Input: dimensioned drawing with shaded views. Units: mm. Origin: part minimum x, y, z. Give positions to 0.01 mm unless a question says otherwise; leave off trailing zeros. Loops run counter-clockwise (first coordinate to the right, second up) from the corner with the lowest first, then second, coordinate; pieces in that order, holes last. Notation, with made-up numbers: (52, -26) -> (106, -26) arc R19 cw to (106, -3) -> close; hole circle Ø11 at (-31.5, 21.25). An arc over 180 degrees is marked (long way). Answer in a Markdown table with one row per item. Add a question column.
1) First-contact query: P1, Ø1.5, axis at y = 12, z = 20, coming from the +X side; P2, Ø0.9, axis at x = 17, z = 28, coming from the -Y side; P3, Ø1, axis at x = 17, z = 9.5, coming from the +Y side. Flat tips, straight axial feed; report the tip coordinate or a pass-through.
2) Line query: line 1 (X direction, y = 15, z = 17) (3 decimals); line 2 (X direction, y = 1.75, z = 16.8); line 3 (X direction, y = 5.25, z = 18). Output: solid intervals per line, ascending. Write a range as from..to.
3) Section query C-C (y = 2). Return the cut outline in (x, z), plus the area to 3 significant figures.
4) Section query A-A (x = 16.8). Return the cut outline in (y, z).
5) Section query D-D (z = 28.05). Return the cut outline in (x, y), plus the area to 3 significant figures.
6) Section query B-B (z = 16.8). Return the cut outline in (x, y), plus the area to 3 significant figures.
7) Draft query along X for the marked faces 1, 2 and 3. Return one class per face: +X half, -X half, draft (parallel to the pull), parting line (faces both ways), or undercut.
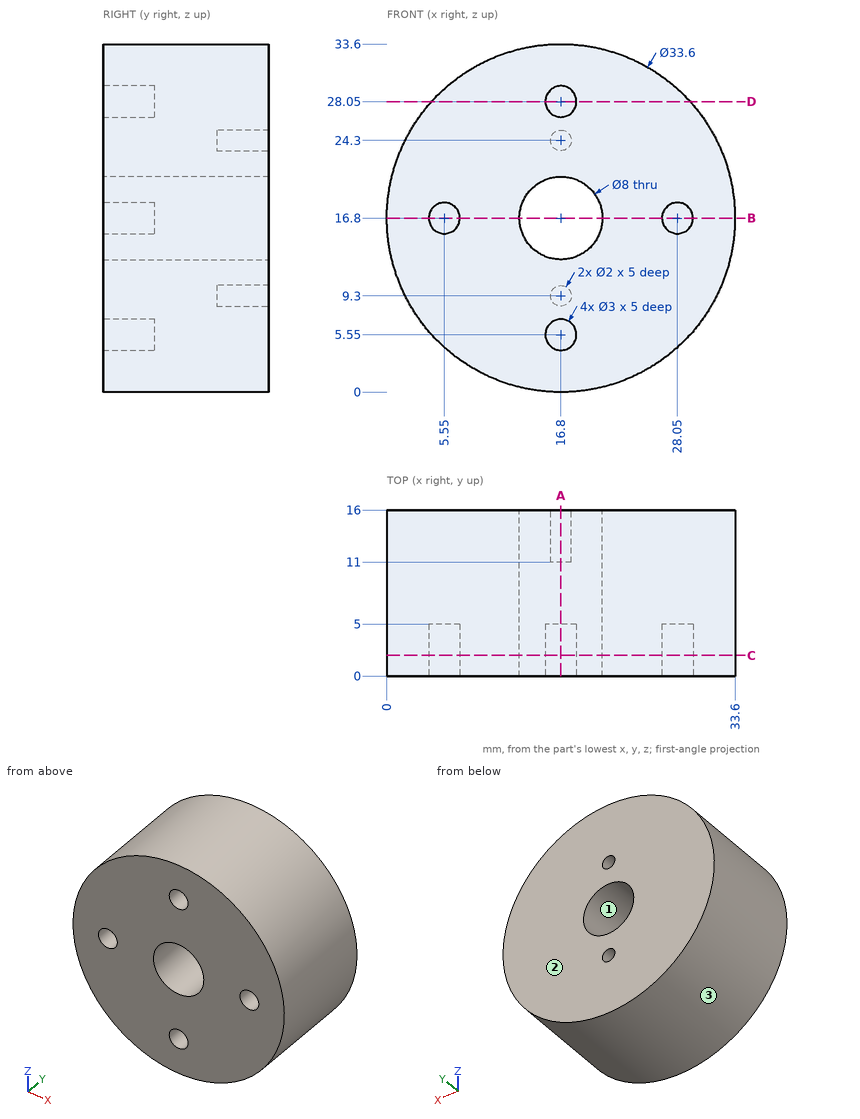
Evaluation:
| question | item | result |
|---|---|---|
| 1 | P1 | x = 33.42 |
| 1 | P2 | y = 5 |
| 1 | P3 | y = 11 |
| 2 | line 1 | 0.001..12.805, 20.795..33.599 |
| 2 | line 2 | 0..4.05, 7.05..12.8, 20.8..26.55, 29.55..33.6 |
| 2 | line 3 | 0.04..12.98, 20.62..33.56 |
| 3 | outline | circle Ø33.6 at (16.8, 16.8); hole circle Ø3 at (5.55, 16.8); hole circle Ø8 at (16.8, 16.8); hole circle Ø3 at (16.8, 5.55); hole circle Ø3 at (16.8, 28.05); hole circle Ø3 at (28.05, 16.8) |
| 3 | area | 808 mm² |
| 4 | outline | (0, 0) -> (16, 0) -> (16, 8.3) -> (11, 8.3) -> (11, 10.3) -> (16, 10.3) -> (16, 12.8) -> (0, 12.8) -> (0, 7.05) -> (5, 7.05) -> (5, 4.05) -> (0, 4.05) -> close; (0, 20.8) -> (16, 20.8) -> (16, 23.3) -> (11, 23.3) -> (11, 25.3) -> (16, 25.3) -> (16, 33.6) -> (0, 33.6) -> (0, 29.55) -> (5, 29.55) -> (5, 26.55) -> (0, 26.55) -> close |
| 5 | outline | (4.32, 0) -> (15.3, 0) -> (15.3, 5) -> (18.3, 5) -> (18.3, 0) -> (29.28, 0) -> (29.28, 16) -> (4.32, 16) -> close |
| 5 | area | 384 mm² |
| 6 | outline | (0, 0) -> (4.05, 0) -> (4.05, 5) -> (7.05, 5) -> (7.05, 0) -> (12.8, 0) -> (12.8, 16) -> (0, 16) -> close; (20.8, 0) -> (26.55, 0) -> (26.55, 5) -> (29.55, 5) -> (29.55, 0) -> (33.6, 0) -> (33.6, 16) -> (20.8, 16) -> close |
| 6 | area | 380 mm² |
| 7 | face 1 | undercut |
| 7 | face 2 | draft |
| 7 | face 3 | parting line |
